```python
from build123d import *

# Parameters (mm, degrees)
SKETCH_W                = 65
SKETCH_H                = 39
PAD_DEPTH               = 1.4
SKETCH001_R             = 1.75
POCKET_DEPTH            = 153.031604
SKETCH001_MIRRORED_2_R  = 1.75
POCKET_MIRRORED_2_DEPTH = 153.031604
SKETCH002_W             = 7.6
SKETCH002_H             = 10
PAD001_DEPTH            = 10
POCKET001_DEPTH         = 5
SKETCH004_W             = 22.6
SKETCH004_H             = 14
PAD002_DEPTH            = 7.5
SKETCH005_R             = 4
PAD003_DEPTH            = 10
SKETCH006_W             = 12
SKETCH006_H             = 12
PAD004_DEPTH            = 7.5
SKETCH007_W             = 9.5
SKETCH007_H             = 4.4
PAD005_DEPTH            = 10
SKETCH008_W             = 10
SKETCH008_H             = 8.4
PAD006_DEPTH            = 4


with BuildPart() as part:
    # Sketch → Pad (new body)
    with BuildSketch(Plane.XY):
        Rectangle(SKETCH_W, SKETCH_H)
    extrude(amount=PAD_DEPTH)

    # Sketch001 → Pocket (cut, through all)
    with BuildSketch(Plane.XY):
        with Locations((29, 16)):
            Circle(SKETCH001_R)
    pocket = extrude(amount=POCKET_DEPTH, mode=Mode.SUBTRACT)

    # Sketch001 Mirrored 2 → Pocket Mirrored 2 (cut, through all)
    with BuildSketch(Plane(origin=(0, 0, 0), x_dir=(-1, 0, 0), z_dir=(0, 0, -1))):
        with Locations((29, 16)):
            Circle(SKETCH001_MIRRORED_2_R)
    pocket_mirrored_2 = extrude(amount=-POCKET_MIRRORED_2_DEPTH, mode=Mode.SUBTRACT)

    # Mirrored001: Pocket, Pocket Mirrored 2 across Sketch001 H_Axis
    add(pocket.mirror(Plane.ZX), mode=Mode.SUBTRACT)
    add(pocket_mirrored_2.mirror(Plane.ZX), mode=Mode.SUBTRACT)

    # Sketch002 → Pad001 (join)
    with BuildSketch(Plane(origin=(0, 0, 0), x_dir=(-1, 0, 0), z_dir=(0, 0, -1))):
        with Locations((-26.7, 0)):
            Rectangle(SKETCH002_W, SKETCH002_H)
    pad001 = extrude(amount=PAD001_DEPTH)

    # Sketch003 → Pocket001 (cut, symmetric)
    with BuildSketch(Plane.XZ):
        Polygon((22.9, -7), (24.9, -10), (22.9, -10), align=None)
        Polygon((29.9, -10), (30.5, -6.159395), (30.5, -10), align=None)
    pocket001 = extrude(amount=POCKET001_DEPTH, both=True, mode=Mode.SUBTRACT)

    # Sketch004 → Pad002 (join)
    with BuildSketch(Plane(origin=(0, 0, 0), x_dir=(-1, 0, 0), z_dir=(0, 0, -1))):
        with Locations((0, -10)):
            Rectangle(SKETCH004_W, SKETCH004_H)
    extrude(amount=PAD002_DEPTH)

    # Sketch005 → Pad003 (join)
    with BuildSketch(Plane(origin=(0, 0, 0), x_dir=(-1, 0, 0), z_dir=(0, 0, -1))):
        with Locations((-20, 11.5)):
            Circle(SKETCH005_R)
    pad003 = extrude(amount=PAD003_DEPTH)

    # Mirrored002: Pad001, Pocket001, Pad003 across Sketch002 V_Axis
    add(pad001.mirror(Plane(origin=(0, 0, 0), x_dir=(0, 0, -1), z_dir=(-1, 0, 0))))
    add(pocket001.mirror(Plane(origin=(0, 0, 0), x_dir=(0, 0, -1), z_dir=(-1, 0, 0))), mode=Mode.SUBTRACT)
    add(pad003.mirror(Plane(origin=(0, 0, 0), x_dir=(0, 0, -1), z_dir=(-1, 0, 0))))

    # Sketch006 → Pad004 (join)
    with BuildSketch(Plane(origin=(0, 0, 0), x_dir=(-1, 0, 0), z_dir=(0, 0, -1))):
        with Locations((7.5, 5)):
            Rectangle(SKETCH006_W, SKETCH006_H)
    extrude(amount=PAD004_DEPTH)

    # Sketch007 → Pad005 (join)
    with BuildSketch(Plane(origin=(0, 0, 0), x_dir=(-1, 0, 0), z_dir=(0, 0, -1))):
        with Locations((8.75, 15.3)):
            Rectangle(SKETCH007_W, SKETCH007_H)
    extrude(amount=PAD005_DEPTH)

    # Sketch008 → Pad006 (join)
    with BuildSketch(Plane(origin=(0, 0, 0), x_dir=(-1, 0, 0), z_dir=(0, 0, -1))):
        with Locations((-6.5, 11.3)):
            Rectangle(SKETCH008_W, SKETCH008_H)
    extrude(amount=PAD006_DEPTH)


solid = part.part
```
The listing builds one solid part. Answer for the finished solid, in the listing's coordinates (mm). A direction names the side the tool comes from. Coordinates: 2 decimals unless noted, no trailing zeros. Write each loop counter-clockwise with the first axis right and the second up, starting at its lowest first coordinate (ties: lowest second). Pieces come first, ordered by that corner, then holes. Notation, with made-up numbers: (-29, -18) - (-25, -18) arc R19 ccw to (-25, -6) - close; hole circle Ø6 at (75, -21.75). An arc over 180 degrees is marked (long way). Return JSON: item names as keys, results as strings. Group by question number.
Q1. For a pull along X with two mould halves and no side action, classify faces 6 (the flat face through (-32.5, 0, 1)), 7 (the flat face through (0, 0, 1.4)), 8 (the flat face through (-13.5, 15, -5)) as +X half, -X half, draft (parallel to the pull), parting line (faces both ways), or undercut.
Q2. Flat-ended cylindrical pins translate along their axes: pin 1 Ø2 at (x, y) = (13.5, -5.5) entering from -Z; pin 2 Ø3.5 at (y, z) = (15, -5.5) entering from +X; pin 3 Ø1.2 at (x, z) = (7.5, -1.5) entering from +Y; pin 4 Ø4.5 at (y, z) = (10, -1.5) entering from +X. Find the tip coordinate at first contact, or state that the pin passes through.
Q3. The part is cut by section C-C on x = 29. Write down the section's boundary in (y, z).
Q4. Find the intervals of material crossed by line 1 along X through (y, z) = (-16, 1.1); line 2 along Y through (x, z) = (-29, 0.5); line 3 along Y through (x, z) = (-10, -1.75), in increasing order. Write a range as [from, to].
Q5. The part is cut by section D-D on y = -11. Write down the section's boundary in (x, z).
Q6. Which of the six approach directions +Z, -Z, +X, -X, +Y, -Y give full straight-line access (tool end or side, diameter ignored) to faces 1 (the cylindrical face through (22.95, 14.2, -4.93)), 2 (the flat face through (-27, -5, -5)), 3 (the flat face through (-30.5, 0, -3)), 4 (the flat face through (-13.5, 5, -4)), 5 (the flat face through (23.9, 0.1, -8.5))?
Q7. The part is cut by section B-B on y = -16. Write down the section's boundary in (x, z).
Q8. The part is cut by section A-A on z = -5. Write down the section's boundary in (x, y).
Evaluation:
{
 "1": {"face 6": "-X half", "face 7": "draft", "face 8": "undercut"},
 "2": {"pin 1": "stops at z = 0", "pin 2": "stops at x = 23.6", "pin 3": "stops at y = 15.5", "pin 4": "stops at x = 32.5"},
 "3": {"outline": "(-19.5, 0) - (-17.75, 0) - (-17.75, 1.4) - (-19.5, 1.4) - close; (-14.25, 0) - (-5, 0) - (-5, -10) - (5, -10) - (5, 0) - (14.25, 0) - (14.25, 1.4) - (-14.25, 1.4) - close; (17.75, 0) - (19.5, 0) - (19.5, 1.4) - (17.75, 1.4) - close"},
 "4": {"line 1": "x = [-32.5, -30.75], [-27.25, 27.25], [30.75, 32.5]", "line 2": "y = [-19.5, -17.75], [-14.25, 14.25], [17.75, 19.5]", "line 3": "y = [-17, -3], [-1, 11], [13.1, 17.5]"},
 "5": {"outline": "(-32.5, 0) - (-11.3, 0) - (-11.3, -7.5) - (11.3, -7.5) - (11.3, 0) - (32.5, 0) - (32.5, 1.4) - (-32.5, 1.4) - close"},
 "6": {"face 1": "-Z", "face 2": "-Z, -X, -Y", "face 3": "-Z, -X, +Y, -Y", "face 4": "-Z, +Y, -Y", "face 5": "-Z, -Y"},
 "7": {"outline": "(-32.5, 0) - (-30.75, 0) - (-30.75, 1.4) - (-32.5, 1.4) - close; (-27.25, 0) - (-11.3, 0) - (-11.3, -7.5) - (11.3, -7.5) - (11.3, 0) - (27.25, 0) - (27.25, 1.4) - (-27.25, 1.4) - close; (30.75, 0) - (32.5, 0) - (32.5, 1.4) - (30.75, 1.4) - close"},
 "8": {"outline": "(-30.5, -5) - (-22.9, -5) - (-22.9, 5) - (-30.5, 5) - close; circle Ø8 at (-20, 11.5); (-13.5, -1) - (-1.5, -1) - (-1.5, 11) - (-13.5, 11) - close; (-13.5, 13.1) - (-4, 13.1) - (-4, 17.5) - (-13.5, 17.5) - close; (-11.3, -17) - (11.3, -17) - (11.3, -3) - (-11.3, -3) - close; circle Ø8 at (20, 11.5); (22.9, -5) - (30.5, -5) - (30.5, 5) - (22.9, 5) - close"}
}
